Input: part model. Units: mm. Frame: model coordinates. A direction names the side the tool comes from. Coordinates: 2 decimals unless noted, no trailing zeros. Write each loop counter-clockwise with the first axis right and the second up, starting at its lowest first coordinate (ties: lowest second). Pieces come first, ordered by that corner, then holes.
1) Line query: L1, parallel to Z at x = 0, y = 0.8; L2, parallel to Z at x = -1.25, y = 6. Output: solid intervals per line, ascending.
2) Draft query along X for faces 3 (the flat face through (-3.1, 5.54, -1.76)), 4 (the flat face through (6.35, 4, 0)), 5 (the flat face through (-3, 0, 0)). Return one class per face: pulls with the +X half, pulls with the -X half, needs draft (parallel to the pull), parting line crosses it, or undercut.
3) Section query C-C (z = -1.25). Output: boundary loops of the cut face in (x, y), then the cut area to 3 significant figures.
4) Section query A-A (x = 0). Output: boundary loops of the cut face in (y, z), then the cut area to 3 significant figures.
5) Set-up query: faces 1 (the flat face through (2, 3, -2)), 2 (the flat face through (-6.35, 4, 0)). Return all of +Z, -Z, +X, -X, +Y, -Y with unobstructed straight access to the full face (end or side cutting, diameter ignored); none if empty.
6) Section query D-D (z = -3). Output: boundary loops of the cut face in (x, y), then the cut area to 3 significant figures.
7) Pin query (flat end, axial travel): pin 1 Ø2 at (x, z) = (-2, 1.5) entering from +Y. Return the tip coordinate at first contact, or that it passes through.
Autodesk Inventor part; units mm, degrees
ref_plane "YZ Plane" through (0, 0, 0) normal (1, 0, 0) x (0, 1, 0)
ref_plane "XZ Plane" through (0, 0, 0) normal (0, 1, 0) x (-1, 0, 0)
ref_plane "XY Plane" through (0, 0, 0) normal (0, 0, 1) x (1, 0, 0)
sketch "Sketch1" plane through (0, 0, 0) normal (0, 1, 0) x (-1, 0, 0)
  line L0 (6.35, 6.35) -> (-6.35, 6.35)
  line L1 (-6.35, 6.35) -> (-6.35, -6.35)
  line L2 (-6.35, -6.35) -> (6.35, -6.35)
  line L3 (6.35, -6.35) -> (6.35, 6.35)
  line L4 (6.35, 6.35) -> (-6.35, -6.35) construction
  line L5 (-6.35, 6.35) -> (6.35, -6.35) construction
  circle A0 centre (0, 0) radius 2.2
  dimension "d0" = 12.7
  dimension "d1" = 12.7
  dimension "d2" = 4.4
extrude "Extrusion1" add sketch "Sketch1" along normal blind 8
sketch "Sketch2" plane through (0, 8, 0) normal (0, 1, 0) x (1, 0, 0)
  circle A0 centre (0, 0) radius 4.115 construction
  line L0 (4.115, 0) -> (2.0575, -3.5637)
  line L1 (2.0575, -3.5637) -> (-2.0575, -3.5637)
  line L2 (-2.0575, -3.5637) -> (-4.115, 0)
  line L3 (-4.115, 0) -> (-2.0575, 3.5637)
  line L4 (-2.0575, 3.5637) -> (2.0575, 3.5637)
  line L5 (2.0575, 3.5637) -> (4.115, 0)
  dimension "d5" = 8.23
extrude "Extrusion2" cut sketch "Sketch2" against normal blind 5
properties part number "M4 net well test"
Answer:
1. L1: z = -6.35 to -2.2, 2.2 to 6.35
1. L2: z = -6.35 to -3.56, 3.56 to 6.35
2. face 3: undercut
2. face 4: pulls with the +X half
2. face 5: needs draft
3. outline: (-6.35, 0) - (-1.81, 0) - (-1.81, 3) - (-3.39, 3) - (-3.39, 8) - (-6.35, 8) - close; (1.81, 0) - (6.35, 0) - (6.35, 8) - (3.39, 8) - (3.39, 3) - (1.81, 3) - close
3. area: 56.8 mm2
4. outline: (0, -6.35) - (8, -6.35) - (8, -3.56) - (3, -3.56) - (3, -2.2) - (0, -2.2) - close; (0, 2.2) - (3, 2.2) - (3, 3.56) - (8, 3.56) - (8, 6.35) - (0, 6.35) - close
4. area: 52.8 mm2
5. face 1: +Y
5. face 2: +Z, -Z, -X, +Y, -Y
6. outline: (-6.35, 0) - (6.35, 0) - (6.35, 8) - (2.38, 8) - (2.38, 3) - (-2.38, 3) - (-2.38, 8) - (-6.35, 8) - close
6. area: 77.8 mm2
7. pin 1: stops at y = 3
